```python
from build123d import *

# Parameters (mm, degrees)
SKETCH1_W           = 0.636
SKETCH1_H           = 0.636
BOSS_EXTRUDE1_DEPTH = 2.54
BOSS_EXTRU_1_DEPTH  = 0.64


with BuildPart() as part:
    # Sketch1 → Boss-Extrude1 (new body)
    with BuildSketch(Plane.XZ):
        Polygon((-0.353553391, -2.186446609), (-2.186446609, -2.186446609), (-2.54, -1.832893219), (-2.54, 0), (-2.186446609, 0.353553391), (-0.353553391, 0.353553391), (0, 0), (0, -1.832893219), align=None)
        with Locations((-1.27, -0.916446609)):
            Rectangle(SKETCH1_W, SKETCH1_H, mode=Mode.SUBTRACT)
    extrude(amount=-BOSS_EXTRUDE1_DEPTH)

    # Esquisse1 → Boss.-Extru.1 (add)
    with BuildSketch(Plane(origin=(-1.588, 0, 0), x_dir=(0, 0, -1), z_dir=(1, 0, 0))):
        with BuildLine():
            Line((0.598446609, 8.54), (0.598446609, -0.18))
            ThreePointArc((0.598446609, -0.18), (1.037786438, -1.240660172), (2.098446609, -1.68))
            Line((2.098446609, -1.68), (5.488446609, -1.68))
            Line((5.488446609, -1.68), (5.488446609, -1.04))
            Line((5.488446609, -1.04), (2.098446609, -1.04))
            ThreePointArc((2.098446609, -1.04), (1.490334778, -0.788111832), (1.238446609, -0.18))
            Line((1.238446609, -0.18), (1.238446609, 8.54))
            Line((1.238446609, 8.54), (0.598446609, 8.54))
        make_face()
    extrude(amount=BOSS_EXTRU_1_DEPTH)


solid = part.part
```
Input: part model. Units: mm. Frame: model coordinates. A direction names the side the tool comes from. Round coordinates to 2 decimals unless told otherwise and drop trailing zeros. Order: outer loops, then holes, each group sorted by start corner. A loop starts at its lowest first (then second) coordinate and runs counter-clockwise, first axis right, second up. Notation, with made-up numbers: (64, 5) - (120, 5) arc R25 ccw to (120, 28) - close; hole circle Ø4 at (-30.75, 79). An arc over 180 degrees is marked (long way). One line per question, with ' | ' between items. Start each with the question number.
1) Cut plane B-B, the plane x = -1.1. Return the cut outline in (y, z), then the cut area to 3 significant figures.
2) Cut plane A-A, the plane z = -2. Return the cut outline in (x, y).
3) Set-up query: faces 4 (the flat face through (-0.948, -1.2, -3)), 5 (the cylindrical face through (-1.3, -0.8, -1.5)), 6 (the flat face through (-2.54, 1, -1)), 7 (the flat face through (0, 1, -1)), 8 (the flat face through (-1, 1, -2.186)). Return all of +Z, -Z, +X, -X, +Y, -Y with unobstructed straight access to the full face (end or side cutting, diameter ignored); none if empty.
4) Cut plane C-C, the plane y = 2. Return the cut outline in (x, z), then the cut area to 3 significant figures.
5) Ray query, probe 1 along X at (y, z) = (5, -1); probe 2 along Z at (x, y) = (-1.4, 1.5); probe 3 along Y at (x, z) = (-1.3, -1.75). Return the intervals inside material, ascending.
6) Cut plane D-D, the plane z = -1.4. Return the cut outline in (x, y), then the cut area to 3 significant figures.
7) Contact query for flat-ended pins moving along their axis: P1, Ø0.9, axis at x = -1, y = 2, coming from the -Z side; P2, Ø1.8, axis at y = -0.5, z = -3, coming from the -X side; P3, Ø3, axis at y = 1.5, z = -3, coming from the -X side; P4, Ø1.5, axis at y = 0, z = -4.5, coming from the +X side. Output: stop coordinate, or through.
8) Pull-direction query (Y, two-part tool) for faces 1 (the cylindrical face through (-1.3, -1.2, -1)), 2 (the flat face through (-1, 0, 0)), 3 (the flat face through (-1.588, -1.2, -3)); classes: +Y half, -Y half, draft (parallel to the pull), parting line (faces both ways), or undercut.
Worked out:
1) outline: (-1.68, -5.49) - (-1.04, -5.49) - (-1.04, -2.1) arc R0.86 cw to (-0.18, -1.24) - (0, -1.24) - (0, -2.19) - (2.54, -2.19) - (2.54, -1.24) - (8.54, -1.24) - (8.54, -0.6) - (2.54, -0.6) - (2.54, 0.35) - (0, 0.35) - (0, -0.6) - (-0.18, -0.6) arc R1.5 ccw to (-1.68, -2.1) - close | area: 13.8 mm^2
2) outline: (-2.37, 0) - (-0.17, 0) - (-0.17, 2.54) - (-2.37, 2.54) - close; (-1.59, -1.68) - (-0.95, -1.68) - (-0.95, -1.03) - (-1.59, -1.03) - close
3) face 4: +Z, -Z, +X, -Y | face 5: -Z, +X, -X | face 6: +Z, -Z, -X, +Y, -Y | face 7: +Z, -Z, +X, +Y, -Y | face 8: -Z, +X, -X, +Y
4) outline: (-2.54, -1.83) - (-2.19, -2.19) - (-0.35, -2.19) - (0, -1.83) - (0, 0) - (-0.35, 0.35) - (-2.19, 0.35) - (-2.54, 0) - close | area: 6.20 mm^2
5) probe 1: x = -1.59 to -0.95 | probe 2: z = -2.19 to 0.35 | probe 3: y = -1.64 to -0.97, 0 to 2.54
6) outline: (-2.54, 0) - (0, 0) - (0, 2.54) - (-2.54, 2.54) - close; (-1.59, -1.51) - (-0.95, -1.51) - (-0.95, -0.68) - (-1.59, -0.68) - close | area: 6.98 mm^2
7) P1: stops at z = -2.19 | P2: stops at x = -1.59 | P3: stops at x = -2.54 | P4: passes through
8) face 1: -Y half | face 2: undercut | face 3: draft
